For this review, take the finished solid that the model builds, in its own axes (mm). A direction names the side the tool comes from. Give positions to 0.01 mm unless a question says otherwise; leave off trailing zeros. Loops run counter-clockwise (first coordinate to the right, second up) from the corner with the lowest first, then second, coordinate; pieces in that order, holes last.
Autodesk Fusion 360 part; units mm, degrees
sketch "Sketch1" plane through (0, 0, 0) normal (0, 0, 1) x (1, 0, 0)
  circle A0 centre (0, 0) radius 3.1
  circle A1 centre (41, 0) radius 3.1
  circle A2 centre (0, 21) radius 3.1
  circle A3 centre (41, 21) radius 3.1
  line L0 (-5.5, 26.5) -> (46.5, 26.5)
  line L1 (46.5, 26.5) -> (46.5, -5.5)
  line L2 (46.5, -5.5) -> (-5.5, -5.5)
  line L3 (-5.5, -5.5) -> (-5.5, 26.5)
  line L4 (3.75, 21) -> (37.25, 21)
  line L5 (37.25, 21) -> (37.25, 0)
  line L6 (37.25, 0) -> (3.75, 0)
  line L7 (3.75, 0) -> (3.75, 21)
  line L8 (20.5, 26.5) -> (20.5, 21) construction
  line L9 (3.75, 10.5) -> (-5.5, 10.5) construction
  point P0 (20.5, 26.5)
  point P1 (20.5, 21)
  point P2 (-5.5, 10.5)
  point P3 (3.75, 10.5)
  dimension "d1" = 6.2
  dimension "d4" = 41
  dimension "d5" = 21
  dimension "d18" = 5.5
  dimension "d19" = 5.5
  dimension "d20" = 32
  dimension "d21" = 52
  dimension "d22" = 33.5
  dimension "d23" = 21
extrude "Extrude1" add sketch "Sketch1" along normal blind 5
extrude "Extrude2" add sketch "Sketch1" along normal blind 2 contours A0 | A1 | A2 | A3
fillet "Fillet1" radius 3 4 edges at (46.5, 26.5, 2.5) (-5.5, 26.5, 2.5) (46.5, -5.5, 2.5) (-5.5, -5.5, 2.5)
Q1. Consider section C-C on z = 1.2. Give the boundary of the cut face in (x, y).
Answers:
outline: (-5.5, -2.5) arc R3 ccw to (-2.5, -5.5) - (43.5, -5.5) arc R3 ccw to (46.5, -2.5) - (46.5, 23.5) arc R3 ccw to (43.5, 26.5) - (-2.5, 26.5) arc R3 ccw to (-5.5, 23.5) - close; hole (3.75, 0) - (37.25, 0) - (37.25, 21) - (3.75, 21) - close
Q2. Consider section B-B on x = 35. Give the boundary of the cut face in (y, z).
Answers:
outline: (-5.5, 0) - (0, 0) - (0, 5) - (-5.5, 5) - close; (21, 0) - (26.5, 0) - (26.5, 5) - (21, 5) - close
Q3. Machinability: for faces 5 (the cylindrical face through (43.864, 1.187, 3.479)), 6 (the flat face through (-5.5, 10, 2)), 7 (the flat face through (20, 21, 2)), which of the approach directions +Z, -Z, +X, -X, +Y, -Y give a long, thin tool a straight path to every point of the face, cutting with its end or side? Answer none if there is none.
Answers:
face 5: +Z
face 6: +Z, -Z, -X, +Y, -Y
face 7: +Z, -Z
Q4. Mouldability with a two-part tool opening along Y and no side actions: class faces 1 (the flat face through (20.1, 21.4, 0)), 2 (the flat face through (41, 0, 2)), 3 (the cylindrical face through (45.6, -4.64, 2.54)), 4 (the flat face through (3.75, 10, 2)) as +Y half, -Y half, draft (parallel to the pull), parting line (faces both ways), or undercut.
Answers:
face 1: draft
face 2: undercut
face 3: -Y half
face 4: undercut
Q5. For probe 1 along Y at (x, z) = (0, 4.4); probe 2 along Y at (x, z) = (9.5, 2.2); probe 3 along X at (y, z) = (8, 1.2), list the stretches that pass through material, from the lowest coordinate up.
Answers:
probe 1: y = -5.5 to -3.1, 3.1 to 17.9, 24.1 to 26.5
probe 2: y = -5.5 to 0, 21 to 26.5
probe 3: x = -5.5 to 3.75, 37.25 to 46.5
Q6. For pin 1 Ø3 at (x, y) = (41.5, 22) entering from +Z; pin 2 Ø5 at (x, y) = (-0.5, 21.5) entering from +Z; pin 3 Ø5 at (x, y) = (31.5, 16.5) entering from +Z, all flat-tipped, find the tip position at first contact; note any pin that passes through.
Answers:
pin 1: stops at z = 2
pin 2: stops at z = 5
pin 3: passes through
Q7. Consider section D-D on z = 4.45. Give the boundary of the cut face in (x, y), plus the area to 3 significant figures.
Answers:
outline: (-5.5, -2.5) arc R3 ccw to (-2.5, -5.5) - (43.5, -5.5) arc R3 ccw to (46.5, -2.5) - (46.5, 23.5) arc R3 ccw to (43.5, 26.5) - (-2.5, 26.5) arc R3 ccw to (-5.5, 23.5) - close; hole circle Ø6.2 at (0, 0); hole circle Ø6.2 at (0, 21); hole (3.75, 0) - (37.25, 0) - (37.25, 21) - (3.75, 21) - close; hole circle Ø6.2 at (41, 0); hole circle Ø6.2 at (41, 21)
area: 832 mm2
Q8. Consider section A-A on y = 12.5. Give the boundary of the cut face in (x, z).
Answers:
outline: (-5.5, 0) - (3.75, 0) - (3.75, 5) - (-5.5, 5) - close; (37.25, 0) - (46.5, 0) - (46.5, 5) - (37.25, 5) - close
